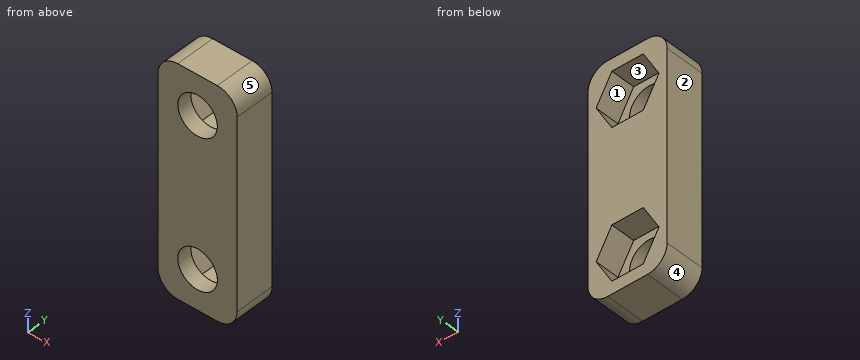
Autodesk Inventor part; units mm, degrees
ref_plane "YZ Plane" through (0, 0, 0) normal (1, 0, 0) x (0, 1, 0)
ref_plane "XZ Plane" through (0, 0, 0) normal (0, 1, 0) x (-1, 0, 0)
ref_plane "XY Plane" through (0, 0, 0) normal (0, 0, 1) x (1, 0, 0)
sketch "Sketch1" plane through (0, 0, 0) normal (0, 1, 0) x (-1, 0, 0)
  line L0 (-4, 11.5) -> (4, 11.5)
  line L1 (4, 11.5) -> (4, -11.5)
  line L2 (4, -11.5) -> (-4, -11.5)
  line L3 (-4, -11.5) -> (-4, 11.5)
  line L4 (-4, 11.5) -> (4, -11.5) construction
  line L5 (4, 11.5) -> (-4, -11.5) construction
  point P0 (0, 0)
  dimension "d0" = 8
  dimension "d1" = 23
extrude "Extrusion1" add sketch "Sketch1" along normal blind 4
sketch "Sketch2" plane through (0, 4, 0) normal (0, 1, 0) x (1, 0, 0)
  line L0 (3.1754, -7.5) -> (1.5877, -10.25)
  line L1 (1.5877, -10.25) -> (-1.5877, -10.25)
  line L2 (-1.5877, -10.25) -> (-3.1754, -7.5)
  line L3 (-3.1754, -7.5) -> (-1.5877, -4.75)
  line L4 (-1.5877, -4.75) -> (1.5877, -4.75)
  line L5 (1.5877, -4.75) -> (3.1754, -7.5)
  line L6 (-4, -11.5) -> (4, -11.5)
  line L7 (-4, 11.5) -> (-4, -11.5)
  line L8 (-4, 0) -> (4, 0)
  line L9 (3.1754, 7.5) -> (1.5877, 10.25)
  line L10 (1.5877, 10.25) -> (-1.5877, 10.25)
  line L11 (-1.5877, 10.25) -> (-3.1754, 7.5)
  line L12 (-3.1754, 7.5) -> (-1.5877, 4.75)
  line L13 (-1.5877, 4.75) -> (1.5877, 4.75)
  line L14 (1.5877, 4.75) -> (3.1754, 7.5)
  point P0 (0, 0)
  point P1 (0, -7.5)
  dimension "d4" = 0
  dimension "d5" = 7.5
  dimension "d6" = 5.5
extrude "Extrusion2" cut sketch "Sketch2" against normal blind 2.5
fillet "Fillet1" radius 2 4 edges at (4, 2, 11.5) (-4, 2, 11.5) (4, 2, -11.5) (-4, 2, -11.5)
sketch "Sketch3" plane through (0, 1.5, 0) normal (0, 1, 0) x (1, 0, 0)
  line L0 (3.1754, -7.5) -> (1.5877, -10.25)
  line L1 (1.5877, -4.75) -> (3.1754, -7.5)
  line L2 (-1.5877, -4.75) -> (1.5877, -4.75)
  line L3 (-3.1754, -7.5) -> (-1.5877, -4.75)
  line L4 (-1.5877, -10.25) -> (-3.1754, -7.5)
  line L5 (1.5877, -10.25) -> (-1.5877, -10.25)
  line L6 (-3.1754, 7.5) -> (-1.5877, 10.25)
  line L7 (-1.5877, 4.75) -> (-3.1754, 7.5)
  line L8 (1.5877, 4.75) -> (-1.5877, 4.75)
  line L9 (3.1754, 7.5) -> (1.5877, 4.75)
  line L10 (1.5877, 10.25) -> (3.1754, 7.5)
  line L11 (-1.5877, 10.25) -> (1.5877, 10.25)
  point P0 (0, 0)
  point P1 (0, -7.5)
  point P2 (0, 7.5)
  dimension "d17" = 2.75
  dimension "d18" = 2.75
hole "Hole1" at (0, 1.5, 7.5) at (0, 1.5, -7.5) direction (0, -1, 0) diameter 4 end through all
properties part number "connector_brace"
Can you work these out from the model? Positions are in its coordinate system, mm. Face numbers are marked on the shaded views. A direction names the side the tool comes from. Give positions to 0.01 mm unless a question says otherwise; leave off trailing zeros. Loops run counter-clockwise (first coordinate to the right, second up) from the corner with the lowest first, then second, coordinate; pieces in that order, holes last. Notation, with made-up numbers: M 63,35.25 L 101,35.25 A8 ccw 101,49.25 Z; hole C 80.25,-0.75 d1. An arc over 180 degrees is marked long. One line per question, with ' | ' between items. Start each with the question number.
Q1. If I drill on line 1 (Z direction, x = 0, y = 0.4); line 2 (X direction, y = 0.55, z = -7.5); line 3 (Z direction, x = -1, y = 1.6), over which ranges is the centre line in solid material (lowest first)? Write a range as from..to.
Q2. For pin 1 Ø3 at (x, z) = (-0.5, -7) entering from +Y, with a flat end and sliding along its axis, tell me the tip position at first contact or that it passes through.
Q3. If we section it at C-C (z = -9): Please give me the cut outline in (x, y).
Q4. If we section it at B-B (y = 2.7): Please give me the cut outline in (x, z).
Q5. For the marked faces 1 and 2, which set-ups out of +Z, -Z, +X, -X, +Y, -Y let a thin tool reach every point of the face, with its end or its side?
Q6. If we mould it in two halves opening along X, with no side actions, what happens to the marked faces 3, 4 and 5? For each: +X half, -X half, draft (parallel to the pull), parting line (faces both ways), or undercut.
Q7. If we section it at A-A (x = 0): Please give me the cut outline in (y, z), plus the area to 3 significant figures.
Computed:
1) line 1: z = -11.5..-9.5, -5.5..5.5, 9.5..11.5 | line 2: x = -4..-2, 2..4 | line 3: z = -11.5..-10.25, -4.75..4.75, 10.25..11.5
2) pin 1: stops at y = 1.5
3) outline: M -4,0 L -1.32,0 L -1.32,1.5 L -2.31,1.5 L -2.31,4 L -4,4 Z; M 1.32,0 L 4,0 L 4,4 L 2.31,4 L 2.31,1.5 L 1.32,1.5 Z
4) outline: M -4,-9.5 A2 ccw -2,-11.5 L 2,-11.5 A2 ccw 4,-9.5 L 4,9.5 A2 ccw 2,11.5 L -2,11.5 A2 ccw -4,9.5 Z; hole M -3.18,-7.5 L -1.59,-10.25 L 1.59,-10.25 L 3.18,-7.5 L 1.59,-4.75 L -1.59,-4.75 Z; hole M -3.18,7.5 L -1.59,4.75 L 1.59,4.75 L 3.18,7.5 L 1.59,10.25 L -1.59,10.25 Z
5) face 1: +Y | face 2: +Z, -Z, -X, +Y, -Y
6) face 3: undercut | face 4: -X half | face 5: +X half
7) outline: M 0,-11.5 L 4,-11.5 L 4,-10.25 L 1.5,-10.25 L 1.5,-9.5 L 0,-9.5 Z; M 0,-5.5 L 1.5,-5.5 L 1.5,-4.75 L 4,-4.75 L 4,4.75 L 1.5,4.75 L 1.5,5.5 L 0,5.5 Z; M 0,9.5 L 1.5,9.5 L 1.5,10.25 L 4,10.25 L 4,11.5 L 0,11.5 Z | area: 52.5 mm²
